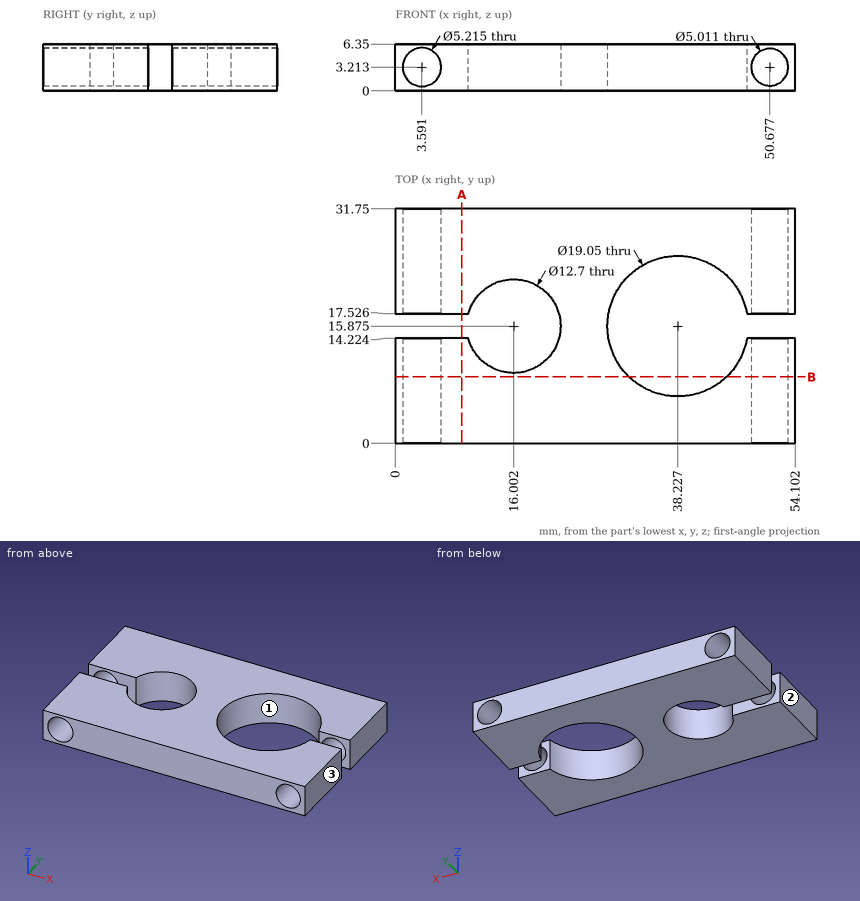
Study the drawing (mm; zero at the part's minimum x, y, z) and answer. Give positions to 0.01 mm unless a question says otherwise; leave off trailing zeros. Loops run counter-clockwise (first coordinate to the right, second up) from the corner with the lowest first, then second, coordinate; pieces in that order, holes last. Notation, with made-up numbers: (-23.5, 54.5) - (28.5, 54.5) arc R21 ccw to (28.5, 67.5) - close; hole circle Ø2 at (61.5, 16). An arc over 180 degrees is marked (long way). Answer in a Markdown table with one row per item. Add a question column.
Q1. The part is cut by section B-B (y = 9). State how many separate pieces and enclosed holes the cut face has, and give its area (3 significant figures).
Q2. Determine the mould class of the marked faces 1, 2 and 3 for opening direction X: released by +X, released by -X, zero draft, split by the parting line, or undercut.
Q3. The part is cut by section A-A (x = 9). Determine the outline of the cut face in (y, z).
Q4. Consider line 1 along X through (y, z) = (26, 3); line 2 along Y through (x, z) = (38.5, 5.5); line 3 along X through (y, z) = (4, 4.25) (1 decimal). Determine where each line is inside the solid, lowest interval first.
Solution:
| question | item | result |
|---|---|---|
| 1 | separate pieces | 2 |
| 1 | enclosed holes | 2 |
| 1 | area | 219 mm² |
| 2 | face 1 | undercut |
| 2 | face 2 | released by -X |
| 2 | face 3 | released by +X |
| 3 | outline | (0, 0) - (14.22, 0) - (14.22, 6.35) - (0, 6.35) - close; (17.53, 0) - (31.75, 0) - (31.75, 6.35) - (17.53, 6.35) - close |
| 4 | line 1 | x = 0 to 0.99, 6.19 to 48.18, 53.17 to 54.1 |
| 4 | line 2 | y = 0 to 6.35, 25.4 to 31.75 |
| 4 | line 3 | x = 0 to 1.2, 6 to 48.4, 53 to 54.1 |
